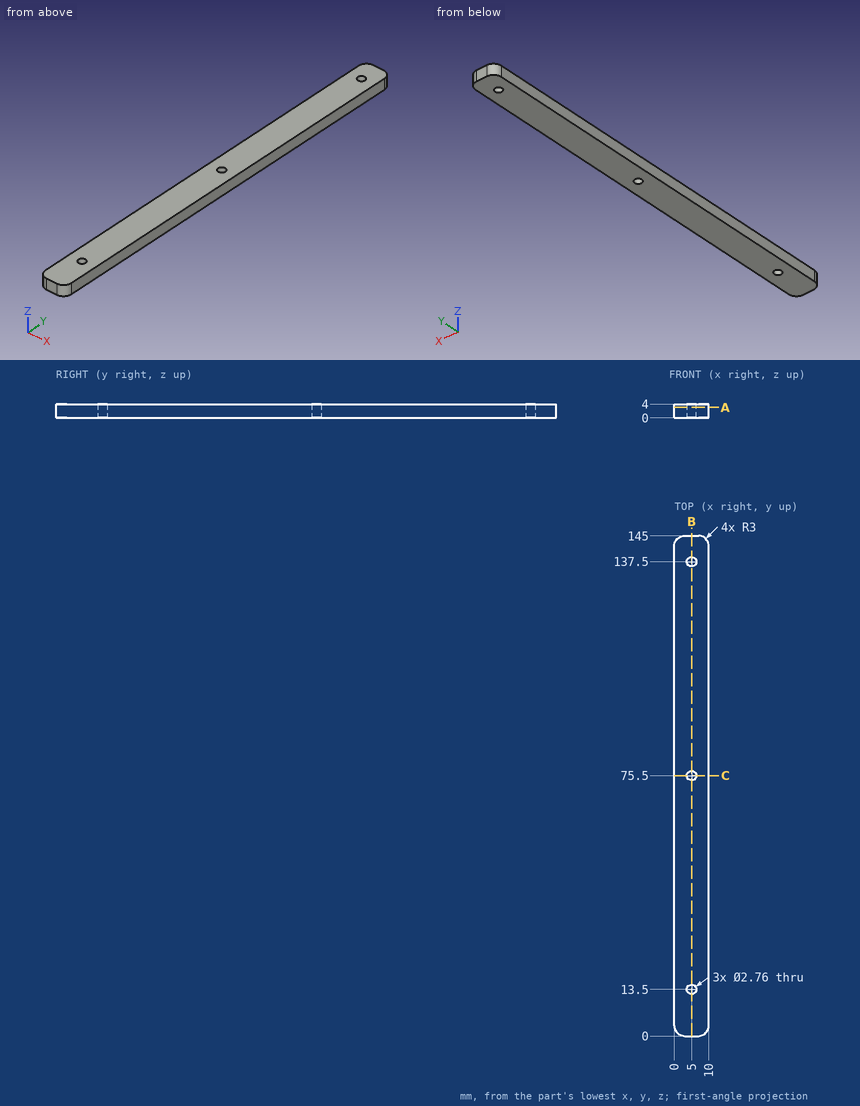
Part print with two shaded views. Sizes in mm from the minimum x, y, z corner. Round coordinates to 2 decimals unless told otherwise and drop trailing zeros. Order: outer loops, then holes, each group sorted by start corner. A loop starts at its lowest first (then second) coordinate and runs counter-clockwise, first axis right, second up. Notation, with made-up numbers: (19, 33.25) - (37, 33.25) arc R17 ccw to (37, 38.25) - close; hole circle Ø10 at (0.25, -10.75). An arc over 180 degrees is marked (long way). Answer in a Markdown table with one row per item. Add a question column.
(1) Probe L1, parallel to Y at x = 5, z = 1.2; L2, parallel to X at y = 137.5, z = 2.05; L3, parallel to Y at x = 3.75, z = 0.85. List the from-to ranges inside material, lowest first. Write a range as [from, to].
(2) Band-saw the part on A-A on z = 3.05. List the corners of the cut face in (x, y), and give its area (3 significant figures).
(3) Drop a flat-ended pin along its axis: pin 1 Ø2.5 at (x, y) = (5, 75.5) entering from -Z. Give the stop position or say it passes through.
(4) Band-saw the part on C-C on y = 75.5. List the corners of the cut face in (x, z), and give its area (3 significant figures).
(5) Band-saw the part on B-B on x = 5. List the corners of the cut face in (y, z).
Data:
| question | item | result |
|---|---|---|
| 1 | L1 | y = [0, 12.12], [14.88, 74.12], [76.88, 136.12], [138.88, 145] |
| 1 | L2 | x = [0, 3.62], [6.38, 10] |
| 1 | L3 | y = [0, 12.92], [14.08, 74.92], [76.08, 136.92], [138.08, 145] |
| 2 | outline | (0, 3) arc R3 ccw to (3, 0) - (7, 0) arc R3 ccw to (10, 3) - (10, 142) arc R3 ccw to (7, 145) - (3, 145) arc R3 ccw to (0, 142) - close; hole circle Ø2.76 at (5, 13.5); hole circle Ø2.76 at (5, 75.5); hole circle Ø2.76 at (5, 137.5) |
| 2 | area | 1,420 mm^2 |
| 3 | pin 1 | passes through |
| 4 | outline | (0, 0) - (3.62, 0) - (3.62, 4) - (0, 4) - close; (6.38, 0) - (10, 0) - (10, 4) - (6.38, 4) - close |
| 4 | area | 29.0 mm^2 |
| 5 | outline | (0, 0) - (12.12, 0) - (12.12, 4) - (0, 4) - close; (14.88, 0) - (74.12, 0) - (74.12, 4) - (14.88, 4) - close; (76.88, 0) - (136.12, 0) - (136.12, 4) - (76.88, 4) - close; (138.88, 0) - (145, 0) - (145, 4) - (138.88, 4) - close |
